Could you check a few things on this model? Use its own coordinates, in mm. Give positions to 0.01 mm unless a question says otherwise; leave off trailing zeros. Order: outer loops, then holes, each group sorted by start corner. A loop starts at its lowest first (then second) coordinate and runs counter-clockwise, first axis right, second up. Notation, with made-up numbers: (45.5, 14) - (77.5, 14) arc R19 ccw to (77.5, 33) - close; hole circle Ø7 at (74, -17.75). An arc over 180 degrees is marked (long way). Put each result on its own line as item: value.
from build123d import *

# Parameters (mm, degrees)
SKETCH2_R           = 1.778
BOSS_EXTRUDE1_DEPTH = 2.54
BOSS_EXTRUDE2_DEPTH = 254


with BuildPart() as part:
    # Sketch2 → Boss-Extrude1 (new body)
    with BuildSketch(Plane.XY):
        with BuildLine():
            Line((-12.7, 0), (-6.35, 0))
            ThreePointArc((-6.35, 0), (0, 6.35), (6.35, 0))
            Line((6.35, 0), (12.7, 0))
            Line((12.7, 0), (12.7, 19.05))
            Line((12.7, 19.05), (-12.7, 19.05))
            Line((-12.7, 19.05), (-12.7, 0))
        make_face()
        with Locations((-8.248891971, 4.7625)):
            Circle(SKETCH2_R, mode=Mode.SUBTRACT)
        with Locations((8.248891971, 4.7625)):
            Circle(SKETCH2_R, mode=Mode.SUBTRACT)
    extrude(amount=BOSS_EXTRUDE1_DEPTH)

    # Sketch3 → Boss-Extrude2 (add)
    with BuildSketch(Plane.XY.offset(2.54)):
        with BuildLine():
            Line((-12.7, 19.05), (-12.7, 13.97))
            Line((-12.7, 13.97), (-3.683, 13.97))
            ThreePointArc((-3.683, 13.97), (-3.323789755, 14.118789755), (-3.175, 14.478))
            Line((-3.175, 14.478), (-3.175, 15.24))
            ThreePointArc((-3.175, 15.24), (-2.803025612, 16.138025612), (-1.905, 16.51))
            Line((-1.905, 16.51), (1.905, 16.51))
            ThreePointArc((1.905, 16.51), (2.803025612, 16.138025612), (3.175, 15.24))
            Line((3.175, 15.24), (3.175, 14.478))
            ThreePointArc((3.175, 14.478), (3.323789755, 14.118789755), (3.683, 13.97))
            Line((3.683, 13.97), (12.7, 13.97))
            Line((12.7, 13.97), (12.7, 19.05))
            Line((12.7, 19.05), (-12.7, 19.05))
        make_face()
    extrude(amount=BOSS_EXTRUDE2_DEPTH)


solid = part.part
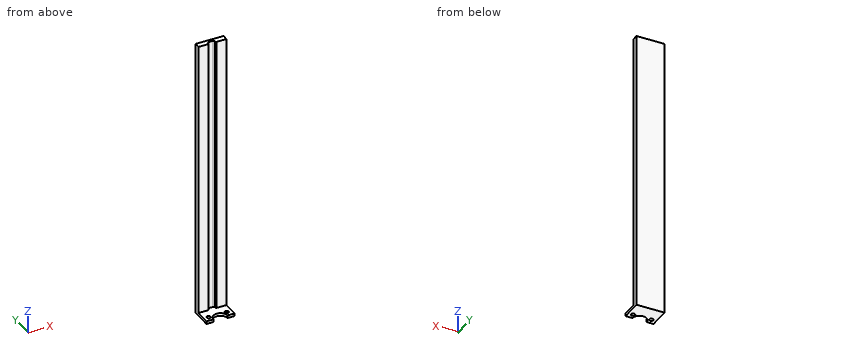
1) If I drill on line 1 (X direction, y = 15.5, z = 36); line 2 (X direction, y = 14.75, z = 86) (3 decimals); line 3 (Z direction, x = 9.75, y = 7), over which ranges is the centre line in solid material (lowest first)? Write a range as [from, to].
Filled in:
line 1: x = [-12.7, -3.15], [3.15, 12.7]
line 2: x = [-12.7, -3.175], [3.175, 12.7]
line 3: z = [0, 2.54]
2) I'm going to push flat-ended pins straight in: pin 1 (5 mm diameter, centred on x = 0.5, y = 6.5, fed in from +Z); pin 2 (2.5 mm diameter, centred on x = -8.5, z = 124.5, fed in from -Y); pin 3 (1.9 mm diameter, centred on x = 0, z = 185.5, fed in from -Y). Where does each tip first touch, or does it pass through?
Filled in:
pin 1: stops at z = 2.54
pin 2: stops at y = 13.97
pin 3: stops at y = 16.51
3) Suppose I cut it at A-A, the plane z = 88. List the corners of the cut face in (x, y) for me (3 decimals), and give its area (3 significant figures).
Filled in:
outline: (-12.7, 13.97) - (-3.683, 13.97) arc R0.508 ccw to (-3.175, 14.478) - (-3.175, 15.24) arc R1.27 cw to (-1.905, 16.51) - (1.905, 16.51) arc R1.27 cw to (3.175, 15.24) - (3.175, 14.478) arc R0.508 ccw to (3.683, 13.97) - (12.7, 13.97) - (12.7, 19.05) - (-12.7, 19.05) - close
area: 113 mm^2
